The figure shows three views and two pictorial views of one solid part (mm, origin at its lowest corner). Answer the questions. A direction names the side the tool comes from. Coordinates: 2 decimals unless noted, no trailing zeros. Loops run counter-clockwise (first coordinate to the right, second up) from the corner with the lowest first, then second, coordinate; pieces in that order, holes last. Notation, with made-up numbers: M 87.25,84 L 128.25,84 A37 ccw 128.25,123 Z; hole C 28.25,26 d3. An arc over 180 degrees is marked long. One line per item, written item: value. Start each with the question number.
1. The part is cut by section C-C (x = 127). Write down the section's boundary in (y, z), then the cut area to 3 significant figures.
2. The part is cut by section B-B (z = 127). Write down the section's boundary in (x, y).
3. For the marked faces 4, 5 and 6, determine the directions among +Z, -Z, +X, -X, +Y, -Y from which every point of the face is accessible in a straight line to the end or side of a thin tool.
4. The part is cut by section A-A (y = 56). Write down the section's boundary in (x, z).
5. The part is cut by section D-D (y = 133). Write down the section's boundary in (x, z).
6. Consider probe 1 along X at (y, z) = (86.5, 93.5); probe 2 along Y at (x, z) = (80, 63); probe 3 along Z at (x, y) = (143.5, 138). Determine where each line is inside the solid, lowest interval first.
7. Determine the mould class of the marked faces 1, 2 and 3 for opening direction X: +X half, -X half, draft (parallel to the pull), parting line (faces both ways), or undercut.
8. Flat-ended cylindrical pins translate along their axes: pin 1 (6.5 mm diameter, centred on x = 148, y = 68.5, fed in from -Z); pin 2 (4 mm diameter, centred on x = 57.5, z = 98.5, fed in from +Y); pin 3 (10 mm diameter, centred on x = 146, y = 75, fed in from +Z). Find the tip coordinate at first contact, or state that the pin passes through.
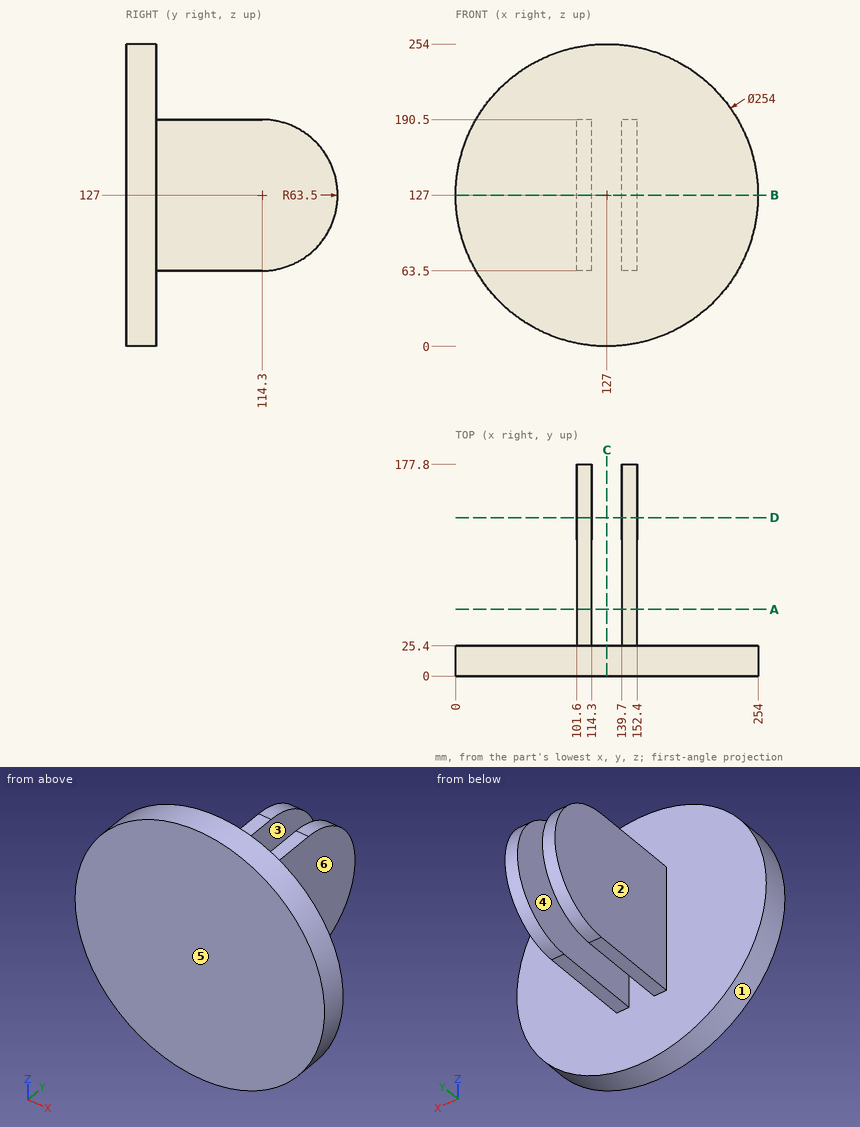
Answer block:
1. outline: M 0,0 L 25.4,0 L 25.4,254 L 0,254 Z
1. area: 6,450 mm2
2. outline: M 0,0 L 254,0 L 254,25.4 L 152.4,25.4 L 152.4,177.8 L 139.7,177.8 L 139.7,25.4 L 114.3,25.4 L 114.3,177.8 L 101.6,177.8 L 101.6,25.4 L 0,25.4 Z
3. face 4: +Z, -Z, +Y
3. face 5: +Z, -Z, +X, -X, -Y
3. face 6: +Z, -Z, +X, +Y
4. outline: M 101.6,63.5 L 114.3,63.5 L 114.3,190.5 L 101.6,190.5 Z; M 139.7,63.5 L 152.4,63.5 L 152.4,190.5 L 139.7,190.5 Z
5. outline: M 101.6,66.32 L 114.3,66.32 L 114.3,187.68 L 101.6,187.68 Z; M 139.7,66.32 L 152.4,66.32 L 152.4,187.68 L 139.7,187.68 Z
6. probe 1: x = 101.6 to 114.3, 139.7 to 152.4
6. probe 2: y = 0 to 25.4
6. probe 3: z = 68.09 to 185.91
7. face 1: parting line
7. face 2: -X half
7. face 3: undercut
8. pin 1: stops at z = 63.5
8. pin 2: stops at y = 25.4
8. pin 3: stops at z = 190.5
